Work out the finished part from the listing and answer in its coordinate system (mm). Face numbers are marked on the shaded views. A direction names the side the tool comes from. Round coordinates to 2 decimals unless told otherwise and drop trailing zeros. Loops run counter-clockwise (first coordinate to the right, second up) from the corner with the lowest first, then second, coordinate; pieces in that order, holes last.
```python
from build123d import *

# Parameters (mm, degrees)
F0_R     = 6.35
F1_DEPTH = 15.24
F2_R     = 11.43
F2_R_2   = 6.35
F3_DEPTH = 12.7


with BuildPart() as f1:
    # F0 (on Front) → F1 (new body)
    with BuildSketch(Plane.XZ):
        Circle(F0_R)
    extrude(amount=F1_DEPTH)

    # F2 (on face) → F3 (join)
    with BuildSketch(Plane.XZ.offset(15.24)):
        Circle(F2_R)
        Circle(F2_R_2, mode=Mode.SUBTRACT)
        Circle(F2_R_2)
    extrude(amount=F3_DEPTH)

    # F4: F1 across plane


with BuildPart() as f1_1:
    add(f1.part)
    add(f1.part.mirror(Plane.XZ))


solid = f1_1.part
```
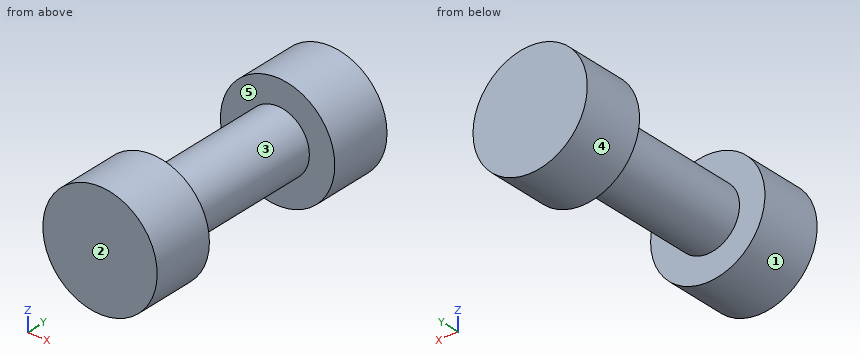
1. Find section A-A (z = 10). Write down the section's boundary in (x, y).
Answer key:
outline: (-5.54, -27.94) - (5.54, -27.94) - (5.54, -15.24) - (-5.54, -15.24) - close; (-5.54, 15.24) - (5.54, 15.24) - (5.54, 27.94) - (-5.54, 27.94) - close
2. Given pin 1 (4 mm diameter, centred on x = -7.5, y = 9, fed in from +Z); pin 2 (2 mm diameter, centred on x = 5.5, y = 17.5, fed in from +Z); pin 3 (4 mm diameter, centred on x = 1.5, y = -16.5, fed in from -Z); pin 4 (6 mm diameter, centred on x = -5.5, y = 14, fed in from +Z), each flat-ended and moving along its own axis, determine where each tip first touches the part or whether it passes through.
Answer key:
pin 1: stops at z = 3.17
pin 2: stops at z = 10.51
pin 3: stops at z = -11.43
pin 4: stops at z = 11.09
3. Find section D-D (z = 0). Write down the section's boundary in (x, y).
Answer key:
outline: (-11.43, -27.94) - (11.43, -27.94) - (11.43, -15.24) - (6.35, -15.24) - (6.35, 15.24) - (11.43, 15.24) - (11.43, 27.94) - (-11.43, 27.94) - (-11.43, 15.24) - (-6.35, 15.24) - (-6.35, -15.24) - (-11.43, -15.24) - close
4. Which of the six approach directions +Z, -Z, +X, -X, +Y, -Y give full straight-line access (tool end or side, diameter ignored) to the marked faces 4 and 5?
Answer key:
face 4: +Y, -Y
face 5: none
5. Determine the mould class of the marked faces 1, 2 and 3 for opening direction Y: +Y half, -Y half, draft (parallel to the pull), parting line (faces both ways), or undercut.
Answer key:
face 1: draft
face 2: -Y half
face 3: undercut
6. Find section C-C (x = 0). Write down the section's boundary in (y, z).
Answer key:
outline: (-27.94, -11.43) - (-15.24, -11.43) - (-15.24, -6.35) - (15.24, -6.35) - (15.24, -11.43) - (27.94, -11.43) - (27.94, 11.43) - (15.24, 11.43) - (15.24, 6.35) - (-15.24, 6.35) - (-15.24, 11.43) - (-27.94, 11.43) - close
7. Find section B-B (x = -7). Write down the section's boundary in (y, z), then the cut area to 3 significant figures.
Answer key:
outline: (-27.94, -9.04) - (-15.24, -9.04) - (-15.24, 9.04) - (-27.94, 9.04) - close; (15.24, -9.04) - (27.94, -9.04) - (27.94, 9.04) - (15.24, 9.04) - close
area: 459 mm2
8. Consider probe 1 along Y at (x, z) = (10.25, 0.5); probe 2 along Z at (x, y) = (0.5, 17); probe 3 along Z at (x, y) = (0, 3). Determine where each line is inside the solid, lowest interval first.
Answer key:
probe 1: y = -27.94 to -15.24, 15.24 to 27.94
probe 2: z = -11.42 to 11.42
probe 3: z = -6.35 to 6.35
